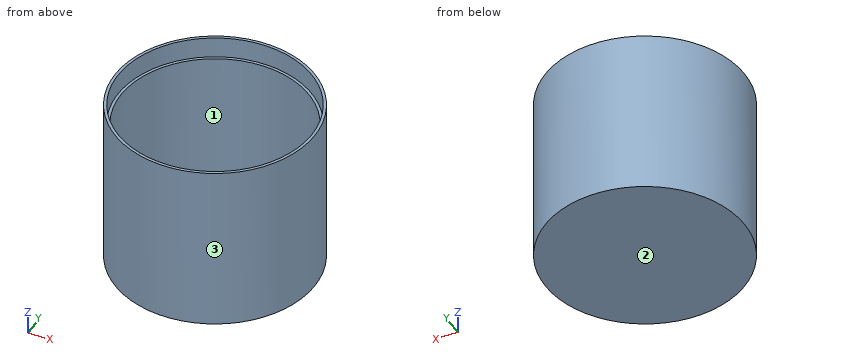
```python
from build123d import *

# Parameters (mm, degrees)
F0_R     = 70
F1_DEPTH = 120
F2_T     = -4
F3_R     = 68
F4_DEPTH = 15


with BuildPart() as f1:
    # F0 (on Top) → F1 (new body)
    with BuildSketch(Plane.XY):
        Circle(F0_R)
    extrude(amount=F1_DEPTH)

    # F2
    f2_openings = [f1.faces().sort_by_distance(p)[0] for p in [
        (0, 0, 120),
    ]]
    offset(amount=F2_T, openings=f2_openings)

    # F3 (on face) → F4 (cut)
    with BuildSketch(Plane.XY.offset(120)):
        Circle(F3_R)
    extrude(amount=-F4_DEPTH, mode=Mode.SUBTRACT)


solid = f1.part
```
Geometry: final body of the model. Coordinates: model frame, mm. Face numbers are marked on the shaded views. Round coordinates to 2 decimals unless told otherwise and drop trailing zeros. Loops run counter-clockwise (first coordinate to the right, second up) from the corner with the lowest first, then second, coordinate; pieces in that order, holes last.
Item 1: Section C-C, the plane z = 25.5. Output: boundary loops of the cut face in (x, y), plus the area to 3 significant figures.
Checked values:
outline: circle Ø140 at (0, 0); hole circle Ø132 at (0, 0)
area: 1,710 mm2
Item 2: Section A-A, the plane x = 0. Output: boundary loops of the cut face in (y, z).
Checked values:
outline: (-70, 0) - (70, 0) - (70, 120) - (68, 120) - (68, 105) - (66, 105) - (66, 4) - (-66, 4) - (-66, 105) - (-68, 105) - (-68, 120) - (-70, 120) - close
Item 3: Line query: L1, parallel to X at y = 1, z = 60.5; L2, parallel to Y at x = 0, z = 65; L3, parallel to Y at x = 0, z = 116.5. Output: solid intervals per line, ascending.
Checked values:
L1: x = -69.99 to -65.99, 65.99 to 69.99
L2: y = -70 to -66, 66 to 70
L3: y = -70 to -68, 68 to 70
Item 4: Mould query, pull axis X, two halves, no side actions, for the marked faces 1, 2 and 3. Classes: released by +X, released by -X, zero draft, split by the parting line, or undercut.
Checked values:
face 1: undercut
face 2: zero draft
face 3: split by the parting line
Item 5: Contact query for flat-ended pins moving along their axis: P1, Ø3, axis at y = -40.5, z = 52, coming from the +X side; P2, Ø10, axis at x = 19, z = 29.5, coming from the +Y side; P3, Ø1, axis at x = 52.5, y = 41.5, coming from the +Z side. Output: stop coordinate, or through.
Checked values:
P1: stops at x = 58.13
P2: stops at y = 68.59
P3: stops at z = 105
